Geometry check sheet. Reference: the model listing, model coordinates, mm. A direction names the side the tool comes from. Coordinates: 2 decimals unless noted, no trailing zeros. Order: outer loops, then holes, each group sorted by start corner. A loop starts at its lowest first (then second) coordinate and runs counter-clockwise, first axis right, second up. Notation, with made-up numbers: (78.25, 77.25) - (88.25, 77.25) arc R13 ccw to (88.25, 102.25) - close; hole circle Ø2 at (1.5, 58). An arc over 180 degrees is marked (long way). Return JSON: item names as keys, results as strings. Group by question number.
Item 1: Section check D-D on y = 42. Enter the section's corners in (x, z).
Item 2: Scan lines: probe 1 along Z at (x, y) = (3, 22); probe 2 along Y at (x, z) = (-0.75, -1.25). Record each from-to range of solid material in increasing order.
Item 3: Section check B-B on z = 1.5. Enter the section's corners in (x, y), then the cut area to 3 significant figures.
Item 4: Gauge pin test, flat end, axial feed: pin 1 (1 mm diameter, centred on x = -2, z = 4, fed in from -Y). Record the tip position at first contact, or that the pin passes through.
Item 5: Section check A-A on y = -30. Enter the section's corners in (x, z), then the cut area to 3 significant figures.
Item 6: Draft check along X on faces 1 (the flat face through (0, 70, 6)), 2 (the cylindrical face through (-0.33, -27.52, 1.48)), 3 (the cylindrical face through (-0.54, 67.56, 4.48)). Enter one of: pulls with the +X half, pulls with the -X half, needs draft (parallel to the pull), parting line crosses it, or undercut.
Item 7: Section check C-C on x = 0. Give the number of separate pieces and of enclosed holes in the cut face, then the cut area to 3 significant figures.
Item 8: Tool access check on faces 4 (the flat face through (0, 80, 1)), 5 (the cylindrical face through (-0.54, 67.56, -1.52)). Record the directions out of +Z, -Z, +X, -X, +Y, -Y that give a thin tool (end or side, any length) a straight path to the whole face; none if there is none.
from build123d import *

# Parameters (mm, degrees)
SKETCH_1_W           = 10
SKETCH_1_H           = 160
SKETCH_1_R           = 2.5
EXTRUDE_1_DEPTH      = 3
EXTRUDE_2_DEPTH      = 3
EXTRUDE_2_DEPTH_BACK = 6
SKETCH_2_R           = 2.5


with BuildPart() as part:
    # 草圖1 → 填料-伸長1 (new body)
    with BuildSketch(Plane.XY):
        Rectangle(SKETCH_1_W, SKETCH_1_H)
        with Locations((0, -70)):
            Circle(SKETCH_1_R, mode=Mode.SUBTRACT)
        with Locations((0, -50)):
            Circle(SKETCH_1_R, mode=Mode.SUBTRACT)
        with Locations((0, -30)):
            Circle(SKETCH_1_R, mode=Mode.SUBTRACT)
        with Locations((0, -10)):
            Circle(SKETCH_1_R, mode=Mode.SUBTRACT)
        with Locations((0, 10)):
            Circle(SKETCH_1_R, mode=Mode.SUBTRACT)
        with Locations((0, 30)):
            Circle(SKETCH_1_R, mode=Mode.SUBTRACT)
        with Locations((0, 50)):
            Circle(SKETCH_1_R, mode=Mode.SUBTRACT)
    extrude(amount=EXTRUDE_1_DEPTH)

    # 草圖2 → 填料-伸長2 (add, two sides: drawn at the far end of the back side and taken through both)
    with BuildSketch(Plane.XY.offset(3).offset(-EXTRUDE_2_DEPTH_BACK)):
        with Locations((0, 70)):
            Circle(SKETCH_2_R)
    extrude(amount=EXTRUDE_2_DEPTH + EXTRUDE_2_DEPTH_BACK)


solid = part.part
Computed:
{
 "1": {"outline": "(-5, 0) - (5, 0) - (5, 3) - (-5, 3) - close"},
 "2": {"probe 1": "z = 0 to 3", "probe 2": "y = 67.62 to 72.38"},
 "3": {"outline": "(-5, -80) - (5, -80) - (5, 80) - (-5, 80) - close; hole circle Ø5 at (0, -70); hole circle Ø5 at (0, -50); hole circle Ø5 at (0, -30); hole circle Ø5 at (0, -10); hole circle Ø5 at (0, 10); hole circle Ø5 at (0, 30); hole circle Ø5 at (0, 50)", "area": "1,460 mm²"},
 "4": {"pin 1": "stops at y = 68"},
 "5": {"outline": "(-5, 0) - (-2.5, 0) - (-2.5, 3) - (-5, 3) - close; (2.5, 0) - (5, 0) - (5, 3) - (2.5, 3) - close", "area": "15.0 mm²"},
 "6": {"face 1": "needs draft", "face 2": "undercut", "face 3": "parting line crosses it"},
 "7": {"separate pieces": "8", "enclosed holes": "0", "area": "405 mm²"},
 "8": {"face 4": "+Z, -Z, +X, -X, +Y", "face 5": "-Z"}
}
